For this review, take the finished solid that the model builds, in its own axes (mm). Face numbers are marked on the shaded views. A direction names the side the tool comes from. Give positions to 0.01 mm unless a question says otherwise; leave off trailing zeros. Write each loop counter-clockwise with the first axis right and the second up, starting at its lowest first coordinate (ties: lowest second). Pieces come first, ordered by that corner, then holes.
1) Draft analysis for pull direction Z (two halves, no side actions). For the marked faces 1, 2 and 3, state which applies: pulls with the +Z half, pulls with the -Z half, needs draft (parallel to the pull), parting line crosses it, or undercut.
2) We need section B-B on z = 9.5. Give the boundary of the cut face in (x, y), and give its area (3 significant figures).
3) Wall thickness on line 1 along Z through (x, y) = (-4, 2.75); line 2 along Z through (x, y) = (-4.75, -3.75); line 3 along Y through (x, z) = (0, 7.75): over which ranges is each line inside the solid? List them lowest first.
4) For P1, Ø3, axis at y = 5, z = 13.5, coming from the +X side; P2, Ø11, axis at x = 0.5, y = -2, coming from the +Z side; P3, Ø4, axis at x = 0.5, y = -0.5, coming from the -Z side; P4, Ø1, axis at y = -6.5, z = 9, coming from the -X side, all flat-tipped, find the tip position at first contact; note any pin that passes through.
5) Machinability: for the marked faces 4, 5, 6 and 7, which of the approach directions +Z, -Z, +X, -X, +Y, -Y give a long, thin tool a straight path to every point of the face, cutting with its end or side? Answer none if there is none.
6) We need section A-A on z = 21. Give the boundary of the cut face in (x, y) (3 decimals).
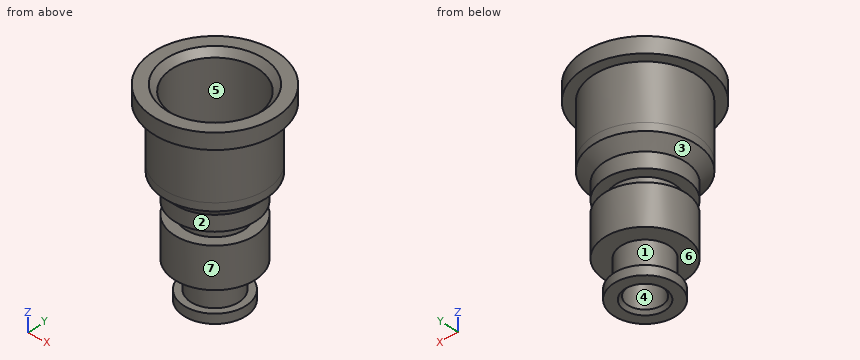
from build123d import *

# Parameters (mm, degrees)
F0_R      = 6.5
F0_R_2    = 2.75
F1_DEPTH  = 20
F2_R      = 6.5
F2_R_2    = 5
F3_DEPTH  = 6
F4_R      = 5
F4_R_2    = 3.875
F5_DEPTH  = 4.5
F7_R      = 6.5
F7_R_2    = 4.75
F8_DEPTH  = 2.032
F9_R      = 8.25
F9_R_2    = 6.5
F10_DEPTH = 3
F11_R     = 8.25
F11_R_2   = 6.875
F12_DEPTH = 11.43
F13_R     = 9.906
F13_R_2   = 8.25
F14_DEPTH = 2.54
F15_SIZE  = 1.74999
F16_SIZE  = 1
F17_SIZE  = 0.5
F18_SIZE  = 1


# Not quite as in the source:
# - a fillet or chamfer is up to 0.001 mm smaller than in the source, because OpenCascade refuses the exact size


with BuildPart() as f1:
    # F0 (on Top) → F1 (new body)
    with BuildSketch(Plane.XY):
        Circle(F0_R)
        Circle(F0_R_2, mode=Mode.SUBTRACT)
    extrude(amount=F1_DEPTH)

    # F2 (on face) → F3 (cut)
    with BuildSketch(Plane(origin=(0, 0, 0), x_dir=(1, 0, 0), z_dir=(0, 0, -1))):
        Circle(F2_R)
        Circle(F2_R_2, mode=Mode.SUBTRACT)
    extrude(amount=-F3_DEPTH, mode=Mode.SUBTRACT)

    # F4 (on face) → F5 (cut)
    with BuildSketch(Plane(origin=(0, 0, 6), x_dir=(1, 0, 0), z_dir=(0, 0, -1))):
        Circle(F4_R)
        Circle(F4_R_2, mode=Mode.SUBTRACT)
    extrude(amount=F5_DEPTH, mode=Mode.SUBTRACT)

    # F7 (on offset) → F8 (cut)
    with BuildSketch(Plane(origin=(0, 0, 12.5), x_dir=(1, 0, 0), z_dir=(0, 0, -1))):
        Circle(F7_R)
        Circle(F7_R_2, mode=Mode.SUBTRACT)
    extrude(amount=-F8_DEPTH, mode=Mode.SUBTRACT)

    # F9 (on face) → F10 (join)
    with BuildSketch(Plane.XY.offset(20)):
        Circle(F9_R)
        Circle(F9_R_2, mode=Mode.SUBTRACT)
    extrude(amount=-F10_DEPTH)

    # F11 (on face) → F12 (join)
    with BuildSketch(Plane.XY.offset(20)):
        Circle(F11_R)
        Circle(F11_R_2, mode=Mode.SUBTRACT)
    extrude(amount=F12_DEPTH)

    # F13 (on face) → F14 (join)
    with BuildSketch(Plane.XY.offset(31.43)):
        Circle(F13_R)
        Circle(F13_R_2, mode=Mode.SUBTRACT)
    extrude(amount=-F14_DEPTH)

    # F15 (size 1.75 in the source; OpenCascade refuses exactly that, so slightly less here)
    f15_edges = [f1.edges().sort_by_distance(p)[0] for p in [
        (-8.25, 0, 17),
    ]]
    chamfer(f15_edges, length=F15_SIZE)

    # F16
    f16_edges = [f1.edges().sort_by_distance(p)[0] for p in [
        (-6.875, 0, 31.43),
    ]]
    chamfer(f16_edges, length=F16_SIZE)

    # F17
    f17_edges = [f1.edges().sort_by_distance(p)[0] for p in [
        (-2.75, 0, 0),
    ]]
    chamfer(f17_edges, length=F17_SIZE)

    # F18
    f18_edges = [f1.edges().sort_by_distance(p)[0] for p in [
        (-2.75, 0, 20),
    ]]
    chamfer(f18_edges, length=F18_SIZE)


solid = f1.part
Results list:
1. face 1: undercut
1. face 2: needs draft
1. face 3: pulls with the -Z half
2. outline: circle Ø13 at (0, 0); hole circle Ø5.5 at (0, 0)
2. area: 109 mm2
3. line 1: z = 0 to 1.5, 6 to 12.5, 14.53 to 20
3. line 2: z = 6 to 12.5, 14.53 to 20
3. line 3: y = -6.5 to -2.75, 2.75 to 6.5
4. P1: stops at x = 5.21
4. P2: stops at z = 31.12
4. P3: passes through
4. P4: stops at x = -2.5
5. face 4: +Z, -Z
5. face 5: +Z
5. face 6: none
5. face 7: -Z
6. outline: circle Ø16.5 at (0, 0); hole circle Ø13.75 at (0, 0)
